Input: part model. Units: mm. Frame: model coordinates. Face numbers are marked on the shaded views. Coordinates: 2 decimals unless noted, no trailing zeros. Loops run counter-clockwise (first coordinate to the right, second up) from the corner with the lowest first, then second, coordinate; pieces in that order, holes last. Notation, with made-up numbers: (69.25, -27.5) -> (77.25, -27.5) arc R21 cw to (77.25, -5.5) -> close; hole circle Ø1 at (60, 11.5). An arc over 180 degrees is marked (long way). Put each result on its own line as item: value. Start each with the question number.
1) Material intervals for L1, parallel to X at y = 28.75, z = -114.5; L2, parallel to Y at x = 44.5, z = -41.5, sorted ascending.
2) Cut plane B-B (y = 28). Return the cut outline in (x, z), plus the area to 3 significant figures.
3) Contact query for flat-ended pins moving along their axis: P1, Ø5, axis at x = 7, z = -140.5, coming from the -Y side; P2, Ø6, axis at x = 47.88, z = -155.57, coming from the +Y side; P3, Ø1.3, axis at x = 51, y = 26.5, coming from the +Z side; P4, Ø1.3, axis at x = 51, y = 23, coming from the -Z side. Output: stop coordinate, or through.
4) Pull-direction query (X, two-part tool) for the marked faces 1 and 2; classes: pulls with the +X half, pulls with the -X half, needs draft (parallel to the pull), parting line crosses it, or undercut.
5) Cut plane D-D (z = -51). Return the cut outline in (x, y), plus the area to 3 significant figures.
6) Cut plane C-C (x = 35). Return the cut outline in (y, z), plus the area to 3 significant figures.
7) Cut plane A-A (y = 21.5). Return the cut outline in (x, z), plus the area to 3 significant figures.
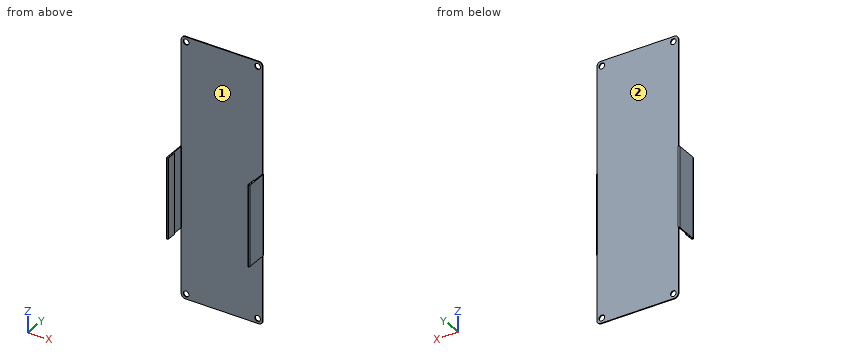
from build123d import *

# Parameters (mm, degrees)
BASE_FLANGE1_DEPTH           = 0.53
M3_CLEARANCE_HOLE1_D         = 3.6
EDGE_FLANGE1_STRIP_W         = 2.6915
EDGE_FLANGE1_STRIP_H         = 0.53
EDGE_FLANGE1_STRIP_CUT_DEPTH = 51.181
EDGE_FLANGE1_DEPTH           = 51.181
HEM1_START                   = -114.74296965
HEM1_DEPTH                   = 51.181
HEM1_2_DEPTH                 = 51.181


# Read off the part's stored shape, not the designer's step: Hem1
# Sheet-metal steps are written as plain solids
with BuildPart() as part:
    # Sketch1 → Base-Flange1 (new body)
    with BuildSketch(Plane(origin=(0, 33.434923007, 0), x_dir=(1, 0, 0), z_dir=(0, 1, 0))):
        with BuildLine():
            Line((1.778, -6.350000017), (25.146, -6.350000017))
            Line((25.146, -6.350000017), (25.146, 76.198203949))
            Line((25.146, 76.198203949), (-0.762, 76.198203949))
            Line((-0.762, 76.198203949), (-0.762, -3.810000017))
            ThreePointArc((-0.762, -3.810000017), (-0.018051224, -5.606051241), (1.778, -6.350000017))
        make_face()
    extrude(amount=BASE_FLANGE1_DEPTH)

    # M3 Clearance Hole1 (through all)
    with Locations(Plane(origin=(0, 33.964923007, 0), x_dir=(1, 0, 0), z_dir=(0, 1, 0))):
        with Locations((2.413, -3.176796068)):
            Hole(M3_CLEARANCE_HOLE1_D / 2)

    # Mirror1: part across plane


with BuildPart() as part_1:
    add(part.part)
    add(part.part.mirror(Plane(origin=(-0.762, 33.964923007, -76.198203949), x_dir=(1, 0, 0), z_dir=(0, 0, 1))))

    # Edge-Flange1 strip (across the edge) → Edge-Flange1 strip cut (cut)
    with BuildSketch(Plane(origin=(-0.6985, 33.434923007, -63.56196965), x_dir=(1, 0, 0), z_dir=(0, 0, -1))):
        with Locations((-1.09175, -0.265)):
            Rectangle(EDGE_FLANGE1_STRIP_W, EDGE_FLANGE1_STRIP_H)
    extrude(amount=EDGE_FLANGE1_STRIP_CUT_DEPTH, mode=Mode.SUBTRACT)

    # Edge-Flange1 section (across the edge) → Edge-Flange1 (add)
    with BuildSketch(Plane(origin=(-0.6985, 33.434923007, -63.56196965), x_dir=(1, 0, 0), z_dir=(0, 0, -1))):
        with BuildLine():
            Line((-0.53, 0.254), (-0.53, 13.97))
            Line((-0.53, 13.97), (0, 13.97))
            Line((0, 13.97), (0, 0.254))
            ThreePointArc((0, 0.254), (0.074394878, 0.074394878), (0.254, 0))
            Line((0.254, 0), (0.254, -0.53))
            ThreePointArc((0.254, -0.53), (-0.300371716, -0.300371716), (-0.53, 0.254))
        make_face()
    extrude(amount=EDGE_FLANGE1_DEPTH)

    # Hem1 outline → Hem1 (cut)
    with BuildSketch(Plane.XY.offset(HEM1_START)):
        with BuildLine():
            Line((-0.6985, 19.464923007), (-0.6985, 19.467082198))
            ThreePointArc((-0.6985, 19.467082198), (-1.075934205, 19.652877091), (-1.2285, 20.044923007))
            Line((-1.2285, 20.044923007), (-1.2285, 19.464923007))
            Line((-1.2285, 19.464923007), (-0.6985, 19.464923007))
        make_face()
    extrude(amount=HEM1_DEPTH, mode=Mode.SUBTRACT)

    # Hem1 2 outline → Hem1 2 (add)
    with BuildSketch(Plane.XY.offset(HEM1_START)):
        with BuildLine():
            Line((-0.0685, 25.814923007), (-0.5985, 25.814923007))
            Line((-0.5985, 25.814923007), (-0.5985, 20.044923007))
            ThreePointArc((-0.5985, 20.044923007), (-0.6485, 19.994923007), (-0.6985, 20.044923007))
            Line((-0.6985, 20.044923007), (-0.6985, 19.467082198))
            ThreePointArc((-0.6985, 19.467082198), (-0.256454084, 19.617488802), (-0.0685, 20.044923007))
            Line((-0.0685, 20.044923007), (-0.0685, 25.814923007))
        make_face()
    extrude(amount=HEM1_2_DEPTH)

    # Mirror2: part across face


with BuildPart() as part_2:
    add(part_1.part)
    add(part_1.part.mirror(Plane(origin=(25.146, 33.699923007, -76.198203949), x_dir=(0, 0, 1), z_dir=(1, 0, 0))))


solid = part_2.part
Results found:
1. L1: x = -1.23 to -0.7, 50.99 to 51.52
1. L2: y = 33.43 to 33.96
2. outline: (-1.23, -114.74) -> (-0.7, -114.74) -> (-0.7, -63.56) -> (-1.23, -63.56) -> close; (50.99, -114.74) -> (51.52, -114.74) -> (51.52, -63.56) -> (50.99, -63.56) -> close
2. area: 54.3 mm2
3. P1: stops at y = 33.43
3. P2: stops at y = 33.96
3. P3: stops at z = -63.56
3. P4: stops at z = -114.74
4. face 1: undercut
4. face 2: needs draft
5. outline: (-0.76, 33.43) -> (51.05, 33.43) -> (51.05, 33.96) -> (-0.76, 33.96) -> close
5. area: 27.5 mm2
6. outline: (33.43, -158.75) -> (33.96, -158.75) -> (33.96, 6.35) -> (33.43, 6.35) -> close
6. area: 87.5 mm2
7. outline: (-1.23, -114.74) -> (-0.7, -114.74) -> (-0.7, -63.56) -> (-1.23, -63.56) -> close; (-0.6, -114.74) -> (-0.07, -114.74) -> (-0.07, -63.56) -> (-0.6, -63.56) -> close; (50.36, -114.74) -> (50.89, -114.74) -> (50.89, -63.56) -> (50.36, -63.56) -> close; (50.99, -114.74) -> (51.52, -114.74) -> (51.52, -63.56) -> (50.99, -63.56) -> close
7. area: 109 mm2
